from build123d import *

# Parameters (mm, degrees)
BOSS_EXTRUDE1_DEPTH      = 150
BOSS_EXTRUDE1_DEPTH_BACK = 150
SKETCH1_R                = 250
SKETCH2_R                = 230
CUT_EXTRUDE2_DEPTH       = 10
SKETCH3_R                = 220
CUT_EXTRUDE3_DEPTH       = 5
FILLET1_R                = 10
FILLET2_R                = 10
SKETCH4_R                = 50
BOSS_EXTRUDE2_DEPTH      = 5
SKETCH5_R                = 42.5
BOSS_EXTRUDE3_DEPTH      = 70
BOSS_EXTRUDE4_START      = 5
SKETCH6_R                = 50
BOSS_EXTRUDE4_DEPTH      = 5
FILLET3_R                = 10
SCALE1_SCALE             = 0.8


# Some blends are built 0.0001 mm under size
with BuildPart() as part:
    # Sketch1 → Boss-Extrude1 (new, two sides: drawn at the far end of the back side and taken through both)
    with BuildSketch(Plane.XY.offset(-BOSS_EXTRUDE1_DEPTH_BACK)):
        Circle(SKETCH1_R)
    extrude(amount=BOSS_EXTRUDE1_DEPTH + BOSS_EXTRUDE1_DEPTH_BACK)

    # Sketch2 → Cut-Extrude2 (cut)
    with BuildSketch(Plane.XY.offset(150)):
        Circle(SKETCH2_R)
    extrude(amount=-CUT_EXTRUDE2_DEPTH, mode=Mode.SUBTRACT)

    # Sketch3 → Cut-Extrude3 (cut)
    with BuildSketch(Plane.XY.offset(140)):
        Circle(SKETCH3_R)
    extrude(amount=-CUT_EXTRUDE3_DEPTH, mode=Mode.SUBTRACT)

    # Fillet1
    fillet1_edges = [part.edges().sort_by_distance(p)[0] for p in [
        (-230, 0, 140),
    ]]
    fillet(fillet1_edges, radius=FILLET1_R - 0.0001)  # a hair under: the kernel refuses the full size

    # Fillet2
    # the kernel refuses this fillet: 10 mm, written as the material it adds along each edge
    with BuildSketch(Plane(origin=(0, 0, 135), x_dir=(1, 0, 0), z_dir=(0, -1, 0))) as fillet2_piece_1:
        with BuildLine():
            CenterArc((211.339745962, 10), FILLET2_R, 270, 60)
            Line((211.339745962, 0), (211.339745962, -0.2))
            Line((211.339745962, -0.2), (220, -0.2))
            Line((220, -0.2), (220.2, 0))
            ThreePointArc((220.2, 0), (220.2, 2.5), (220.173205081, 4.9))
            Line((220.173205081, 4.9), (220, 5))
        make_face()
    revolve(axis=Axis((0, 0, 135), (0, 0, 1)))

    # Sketch4 → Boss-Extrude2 (add)
    with BuildSketch(Plane.XY.offset(135)):
        Circle(SKETCH4_R)
    extrude(amount=BOSS_EXTRUDE2_DEPTH)

    # Sketch5 → Boss-Extrude3 (add)
    with BuildSketch(Plane.XY.offset(140)):
        Circle(SKETCH5_R)
    extrude(amount=BOSS_EXTRUDE3_DEPTH)

    # Sketch6 → Boss-Extrude4 (add)
    with BuildSketch(Plane(origin=(0, 0, -150), x_dir=(-1, 0, 0), z_dir=(0, 0, -1)).offset(BOSS_EXTRUDE4_START)):
        with Locations(Location((0, 0, 0), (0, 0, 180))):
            Circle(SKETCH6_R)
    extrude(amount=-BOSS_EXTRUDE4_DEPTH)

    # Fillet3
    # the kernel refuses this fillet: 10 mm, written as the material it adds along each edge
    with BuildSketch(Plane(origin=(0, 0, 135), x_dir=(1, 0, 0), z_dir=(0, -1, 0))) as fillet3_piece_1:
        with BuildLine():
            CenterArc((58.660254038, 10), FILLET3_R, 210, 60)
            Line((50, 5), (49.826794919, 4.9))
            ThreePointArc((49.826794919, 4.9), (49.8, 2.5), (49.8, 0))
            Line((49.8, 0), (50, -0.2))
            Line((50, -0.2), (58.660254038, -0.2))
            Line((58.660254038, -0.2), (58.660254038, 0))
        make_face()
    revolve(axis=Axis((0, 0, 135), (0, 0, 1)))
    with BuildSketch(Plane(origin=(0, 0, 140), x_dir=(1, 0, 0), z_dir=(0, -1, 0))) as fillet3_piece_2:
        with BuildLine():
            CenterArc((52.5, 9.682458366), FILLET3_R, 180, 75.522487814)
            Line((42.5, 9.682458366), (42.3, 9.682458366))
            Line((42.3, 9.682458366), (42.3, 0))
            Line((42.3, 0), (42.5, -0.2))
            ThreePointArc((42.5, -0.2), (46.25, -0.2), (49.95, -0.193649167))
            Line((49.95, -0.193649167), (50, 0))
        make_face()
    revolve(axis=Axis((0, 0, 140), (0, 0, 1)))


with BuildPart() as part_1:
    # Scale1: scaled about (0, 0, -4.710262046)
    add(part.part.scale(SCALE1_SCALE).moved(Location((0, 0, -0.942052409))))


solid = part_1.part
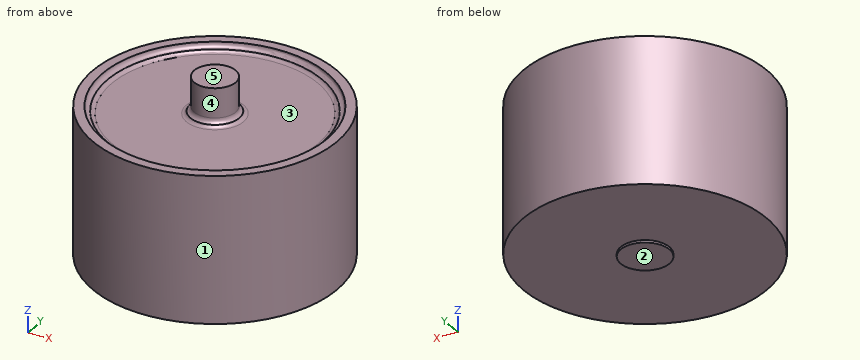
The model under review builds one solid part; all positions refer to its coordinate system, in mm. Face numbers are marked on the shaded views. A direction names the side the tool comes from. Coordinates: 2 decimals unless noted, no trailing zeros. Loops run counter-clockwise (first coordinate to the right, second up) from the corner with the lowest first, then second, coordinate; pieces in that order, holes last. Notation, with made-up numbers: (45, 1.25) -> (87, 1.25) arc R15 cw to (87, 10.25) -> close; hole circle Ø6 at (-14, -18). An arc over 180 degrees is marked (long way). Use a Markdown table: item, result. Add a question column.
1. Machinability: for the marked faces 4 and 5, which of the approach directions +Z, -Z, +X, -X, +Y, -Y give a long, thin tool a straight path to every point of the face, cutting with its end or side? Answer none if there is none.
2. Clearance check with flat-ended pins moving along their axes: pin 1 Ø3 at (y, z) = (-90.5, -0.5) entering from +X; pin 2 Ø6 at (x, y) = (-22, 100) entering from +Z; pin 3 Ø6 at (x, z) = (44, 97.5) entering from -Y; pin 4 Ø2 at (x, z) = (39, 121) entering from +Y. State where each tip first meets the part, or that it passes through.
3. To check wall thickness, follow line 1 (Y direction, x = 0, z = 119); line 2 (Z direction, x = 103.5, y = 77); line 3 (Y direction, x = 0, z = 119.1). State the ranges of each line that lie inside material, in increasing order.
4. Draft analysis for pull direction X (two halves, no side actions). For the marked faces 1, 2 and 3, state which applies: pulls with the +X half, pulls with the -X half, needs draft (parallel to the pull), parting line crosses it, or undercut.
5. Add section C-C on z = -38. Write out the cut boundary in (x, y).
Returned:
| question | item | result |
|---|---|---|
| 1 | face 4 | +Z |
| 1 | face 5 | +Z, +X, -X, +Y, -Y |
| 2 | pin 1 | stops at x = 179.11 |
| 2 | pin 2 | stops at z = 107.06 |
| 2 | pin 3 | stops at y = -195.75 |
| 2 | pin 4 | passes through |
| 3 | line 1 | y = -200 to -184, -34 to 34, 184 to 200 |
| 3 | line 2 | z = -120.94 to 107.06 |
| 3 | line 3 | y = -34 to 34 |
| 4 | face 1 | parting line crosses it |
| 4 | face 2 | needs draft |
| 4 | face 3 | undercut |
| 5 | outline | circle Ø400 at (0, 0) |
